from build123d import *

# Parameters (mm, degrees)
F0_R        = 4.25
F0_R_2      = 2.6
F1_DEPTH    = 10
F0_R_3      = 10.25
F0_R_4      = 1.6
F2_DEPTH    = 10
F3_DEPTH    = 10
F4_DEPTH    = 10
F5_T2_ANGLE = 100.939379093
F5_T4_ANGLE = 100.939379093
F5_T6_ANGLE = 100.939379093
F5_T8_ANGLE = 100.939379093


# Not quite as in the source:
# - a fillet or chamfer that OpenCascade refuses, or shapes differently, is made with other operations: its cross-section is extruded or revolved along the edge and cut away or added


with BuildPart() as f1:
    # F0 (on Top) → F1 (new body)
    with BuildSketch(Plane.XY):
        Circle(F0_R)
        Circle(F0_R_2, mode=Mode.SUBTRACT)
    extrude(amount=F1_DEPTH)

    # F0 (on Top) → F2 (join)
    with BuildSketch(Plane.XY):
        Circle(F0_R_3)
        with Locations((0, -7)):
            Circle(F0_R_2, mode=Mode.SUBTRACT)
        with Locations((-7, 0)):
            Circle(F0_R_4, mode=Mode.SUBTRACT)
        with Locations((-4.95, 4.9494949237)):
            Circle(F0_R_4, mode=Mode.SUBTRACT)
        Circle(F0_R, mode=Mode.SUBTRACT)
        with Locations((4.95, 4.9494949237)):
            Circle(F0_R_4, mode=Mode.SUBTRACT)
        with Locations((7, 0)):
            Circle(F0_R_4, mode=Mode.SUBTRACT)
        with Locations((0, 7)):
            Circle(F0_R_4, mode=Mode.SUBTRACT)
    extrude(amount=F2_DEPTH)

    # F0 (on Top) → F3 (join)
    with BuildSketch(Plane.XY):
        with BuildLine():
            ThreePointArc((11.5318049333, -3.3192581973), (11.8823747458, -1.6760579943), (12, 0))
            ThreePointArc((12, 0), (11.8823747458, 1.6760579943), (11.5318049333, 3.3192581973))
            ThreePointArc((11.5318049333, 3.3192581973), (8.3601945025, 8.6085508583), (2.9803472847, 11.6240066269))
            ThreePointArc((2.9803472847, 11.6240066269), (0, 12), (-2.9803472847, 11.6240066269))
            ThreePointArc((-2.9803472847, 11.6240066269), (-8.3601945025, 8.6085508583), (-11.5318049333, 3.3192581973))
            ThreePointArc((-11.5318049333, 3.3192581973), (-12, 0), (-11.5318049333, -3.3192581973))
            ThreePointArc((-11.5318049333, -3.3192581973), (-8.3601945025, -8.6085508583), (-2.9803472847, -11.6240066269))
            ThreePointArc((-2.9803472847, -11.6240066269), (0, -12), (2.9803472847, -11.6240066269))
            ThreePointArc((2.9803472847, -11.6240066269), (8.3601945025, -8.6085508583), (11.5318049333, -3.3192581973))
        make_face()
        Circle(F0_R_3, mode=Mode.SUBTRACT)
    extrude(amount=F3_DEPTH)

    # F0 (on Top) → F4 (join, symmetric)
    with BuildSketch(Plane.XY):
        with BuildLine():
            ThreePointArc((2.9803472847, 11.6240066269), (8.3601945025, 8.6085508583), (11.5318049333, 3.3192581973))
            Line((11.5318049333, 3.3192581973), (12.9980264072, 3.6470960391))
            ThreePointArc((12.9980264072, 3.6470960391), (9.4466784184, 9.6441830582), (3.3774018659, 13.070698399))
            Line((3.3774018659, 13.070698399), (2.9803472847, 11.6240066269))
        make_face()
        with BuildLine():
            ThreePointArc((-11.5318049333, 3.3192581973), (-8.3601945025, 8.6085508583), (-2.9803472847, 11.6240066269))
            Line((-2.9803472847, 11.6240066269), (-3.3774018659, 13.070698399))
            ThreePointArc((-3.3774018659, 13.070698399), (-9.4466784184, 9.6441830582), (-12.9980264072, 3.6470960391))
            Line((-12.9980264072, 3.6470960391), (-11.5318049333, 3.3192581973))
        make_face()
        with BuildLine():
            Line((-3.3774018659, -13.070698399), (-2.9803472847, -11.6240066269))
            ThreePointArc((-2.9803472847, -11.6240066269), (-8.3601945025, -8.6085508583), (-11.5318049333, -3.3192581973))
            Line((-11.5318049333, -3.3192581973), (-12.9980264072, -3.6470960391))
            ThreePointArc((-12.9980264072, -3.6470960391), (-9.4466784184, -9.6441830582), (-3.3774018659, -13.070698399))
        make_face()
        with BuildLine():
            Line((12.9980264072, -3.6470960391), (11.5318049333, -3.3192581973))
            ThreePointArc((11.5318049333, -3.3192581973), (8.3601945025, -8.6085508583), (2.9803472847, -11.6240066269))
            Line((2.9803472847, -11.6240066269), (3.3774018659, -13.070698399))
            ThreePointArc((3.3774018659, -13.070698399), (9.4466784184, -9.6441830582), (12.9980264072, -3.6470960391))
        make_face()
    extrude(amount=F4_DEPTH, both=True)

    # F5: fillet of radius 2 on 4 edges, made by hand

    # F5_s1 → F5_t2 (revolve, cut)
    with BuildSketch(Plane(origin=(0, 0, 0), x_dir=(0, 0, 1), z_dir=(-0.0850162065, -0.9963795686, 0))):
        with BuildLine():
            ThreePointArc((-10, -12), (-9.2882531983, -13.0811388301), (-8.0635083269, -13.5))
            Line((-8.0635083269, -13.5), (-10, -13.5))
            Line((-10, -13.5), (-10, -12))
        make_face()
    revolve(axis=Axis((0, 0, -10), (0, 0, 1)), revolution_arc=F5_T2_ANGLE, mode=Mode.SUBTRACT)

    # F5_s3 → F5_t4 (revolve, cut)
    with BuildSketch(Plane(origin=(0, 0, 0), x_dir=(0, 0, 1), z_dir=(0.9944074241, -0.1056119072, 0))):
        with BuildLine():
            ThreePointArc((-10, -12), (-9.2882531983, -13.0811388301), (-8.0635083269, -13.5))
            Line((-8.0635083269, -13.5), (-10, -13.5))
            Line((-10, -13.5), (-10, -12))
        make_face()
    revolve(axis=Axis((0, 0, -10), (0, 0, 1)), revolution_arc=F5_T4_ANGLE, mode=Mode.SUBTRACT)

    # F5_s5 → F5_t6 (revolve, cut)
    with BuildSketch(Plane(origin=(0, 0, 0), x_dir=(0, 0, 1), z_dir=(0.0850162065, 0.9963795686, 0))):
        with BuildLine():
            ThreePointArc((-10, -12), (-9.2882531983, -13.0811388301), (-8.0635083269, -13.5))
            Line((-8.0635083269, -13.5), (-10, -13.5))
            Line((-10, -13.5), (-10, -12))
        make_face()
    revolve(axis=Axis((0, 0, -10), (0, 0, 1)), revolution_arc=F5_T6_ANGLE, mode=Mode.SUBTRACT)

    # F5_s7 → F5_t8 (revolve, cut)
    with BuildSketch(Plane(origin=(0, 0, 0), x_dir=(0, 0, 1), z_dir=(-0.9944074241, 0.1056119072, 0))):
        with BuildLine():
            ThreePointArc((-10, -12), (-9.2882531983, -13.0811388301), (-8.0635083269, -13.5))
            Line((-8.0635083269, -13.5), (-10, -13.5))
            Line((-10, -13.5), (-10, -12))
        make_face()
    revolve(axis=Axis((0, 0, -10), (0, 0, 1)), revolution_arc=F5_T8_ANGLE, mode=Mode.SUBTRACT)


solid = f1.part
Can you work these out from the model? Positions are in its coordinate system, mm. A direction names the side the tool comes from. Coordinates: 2 decimals unless noted, no trailing zeros. Order: outer loops, then holes, each group sorted by start corner. A loop starts at its lowest first (then second) coordinate and runs counter-clockwise, first axis right, second up. Notation, with made-up numbers: M -15,75 L 30,75 A14 ccw 30,82 Z; hole C 85,-33.75 d11. An arc over 180 degrees is marked long. Write item = value, one per line.
(1) Suppose I cut it at C-C on z = 1.75. Please give me the cut outline in (x, y).
Results are:
outline = M -13,-3.65 A13.5 ccw -3.38,-13.07 L -2.98,-11.62 A12 ccw 2.98,-11.62 L 3.38,-13.07 A13.5 ccw 13,-3.65 L 11.53,-3.32 A12 ccw 11.53,3.32 L 13,3.65 A13.5 ccw 3.38,13.07 L 2.98,11.62 A12 ccw -2.98,11.62 L -3.38,13.07 A13.5 ccw -13,3.65 L -11.53,3.32 A12 ccw -11.53,-3.32 Z; hole C -7,0 d3.2; hole C -4.95,4.95 d3.2; hole C 0,-7 d5.2; hole C 0,0 d5.2; hole C 0,7 d3.2; hole C 4.95,4.95 d3.2; hole C 7,0 d3.2
(2) If we mould it in two halves opening along Y, with no side actions, what happens to faces 5 (the face through (0, -3, 10)), 6 (the face through (-0.338, -4.422, 4.93)), 7 (the face through (9.38, -9.71, 1.09))? For each: pulls with the +Y half, pulls with the -Y half, needs draft (parallel to the pull), parting line crosses it, or undercut.
Results are:
face_5 = needs draft
face_6 = undercut
face_7 = pulls with the -Y half
(3) For faces 1 (the face through (8.42, -8.55, -4.93)), 2 (the face through (3.176, -12.337, 0.14)), 3 (the face through (12.275, -3.485, 0.14)), 4 (the face through (-12.275, 3.485, -0.14)), which set-ups out of +Z, -Z, +X, -X, +Y, -Y let a thin tool reach every point of the face, with its end or its side?
Results are:
face_1 = -Z
face_2 = +Z, -Z, -Y
face_3 = +Z, -Z, +X
face_4 = +Z, -Z, -X
(4) Suppose I cut it at B-B on z = -2.5. Please give me the cut outline in (x, y), plus the area to 3 significant figures.
Results are:
outline = M -13,-3.65 A13.5 ccw -3.38,-13.07 L -2.98,-11.62 A12 cw -11.53,-3.32 Z; M -13,3.65 L -11.53,3.32 A12 cw -2.98,11.62 L -3.38,13.07 A13.5 ccw Z; M 2.98,-11.62 L 3.38,-13.07 A13.5 ccw 13,-3.65 L 11.53,-3.32 A12 cw Z; M 2.98,11.62 A12 cw 11.53,3.32 L 13,3.65 A13.5 ccw 3.38,13.07 Z
area = 79.7 mm2
(5) I need wall thicknesses on line 1 along Y through (x, z) = (0, 3.5); line 2 along Y through (x, z) = (-1, 7); line 3 along Z through (x, y) = (-5.75, 1.25). Which ranges of each line are inside material? Lowest first, please. Write a range as [from, to].
Results are:
line_1 = [-12, -9.6], [-4.4, -2.6], [2.6, 5.4], [8.6, 12]
line_2 = [-11.96, -9.4], [-4.6, -2.4], [2.4, 5.75], [8.25, 11.96]
line_3 = [0, 10]
(6) For pin 1 Ø8.5 at (x, y) = (0, -7) entering from -Z; pin 2 Ø1 at (y, z) = (2.5, 8) entering from +X; pin 3 Ø6 at (y, z) = (-3.5, -1.5) entering from -X; pin 4 Ø3 at (x, y) = (-4.95, 4.95) entering from +Z, each with a flat end and sliding along its axis, tell me the tip position at first contact or that it passes through.
Results are:
pin_1 = 0
pin_2 = 11.83
pin_3 = -13
pin_4 = through
(7) Suppose I cut it at A-A on x = 0. Please give me the cut outline in (y, z), plus the area to 3 significant figures.
Results are:
outline = M -12,0 L -9.6,0 L -9.6,10 L -12,10 Z; M -4.4,0 L -2.6,0 L -2.6,10 L -4.4,10 Z; M 2.6,0 L 5.4,0 L 5.4,10 L 2.6,10 Z; M 8.6,0 L 12,0 L 12,10 L 8.6,10 Z
area = 104 mm2
